Autodesk Inventor part; units mm, degrees
ref_plane "YZ Plane" through (0, 0, 0) normal (1, 0, 0) x (0, 1, 0)
ref_plane "XZ Plane" through (0, 0, 0) normal (0, 1, 0) x (-1, 0, 0)
ref_plane "XY Plane" through (0, 0, 0) normal (0, 0, 1) x (1, 0, 0)
sketch "Sketch1" plane through (0, 0, 0) normal (0, 0, 1) x (1, 0, 0)
  line L0 (0, 0) -> (0, 10)
  line L1 (0, 10) -> (-3, 10)
  line L2 (-3, 10) -> (-3, 20)
  line L3 (-3, 20) -> (0, 20)
  line L4 (0, 20) -> (0, 30)
  line L5 (0, 30) -> (38.5, 30)
  line L6 (38.5, 30) -> (38.5, 33)
  line L7 (38.5, 33) -> (48.5, 33)
  line L8 (48.5, 33) -> (48.5, 30)
  line L9 (48.5, 30) -> (87, 30)
  line L10 (87, 30) -> (87, 20)
  line L11 (87, 20) -> (90, 20)
  line L12 (90, 20) -> (90, 10)
  line L13 (90, 10) -> (87, 10)
  line L14 (87, 10) -> (87, 0)
  line L15 (87, 0) -> (48.5, 0)
  line L16 (48.5, 0) -> (48.5, -3)
  line L17 (48.5, -3) -> (38.5, -3)
  line L18 (38.5, -3) -> (38.5, 0)
  line L19 (38.5, 0) -> (0, 0)
  line L20 (10, 25) -> (20, 25)
  line L21 (25, 20) -> (25, 10)
  line L22 (20, 5) -> (10, 5)
  line L23 (5, 10) -> (5, 20)
  line L24 (67, 25) -> (77, 25)
  line L25 (82, 20) -> (82, 10)
  line L26 (77, 5) -> (67, 5)
  line L27 (62, 10) -> (62, 20)
  arc A0 (10, 25) -> (5, 20) centre (10, 20) ccw
  arc A1 (25, 20) -> (20, 25) centre (20, 20) ccw
  arc A2 (20, 5) -> (25, 10) centre (20, 10) ccw
  arc A3 (5, 10) -> (10, 5) centre (10, 10) ccw
  arc A4 (67, 25) -> (62, 20) centre (67, 20) ccw
  arc A5 (82, 20) -> (77, 25) centre (77, 20) ccw
  arc A6 (77, 5) -> (82, 10) centre (77, 10) ccw
  arc A7 (62, 10) -> (67, 5) centre (67, 10) ccw
  circle A8 centre (43.5, 15) radius 2.5
  circle A9 centre (35.3683, 23.1317) radius 1
  circle A10 centre (35.3683, 6.8683) radius 1
  circle A11 centre (51.6317, 6.8683) radius 1
  circle A12 centre (51.6317, 23.1317) radius 1
  dimension "d0" = 10
  dimension "d1" = 10
  dimension "d2" = 10
  dimension "d3" = 10
  dimension "d4" = 10
  dimension "d5" = 10
  dimension "d6" = 38.5
  dimension "d7" = 38.5
  dimension "d8" = 10
  dimension "d9" = 38.5
  dimension "d11" = 38.5
  dimension "d12" = 5
  dimension "d13" = 5
  dimension "d15" = 5
  dimension "d16" = 20
  dimension "d17" = 5
  dimension "d18" = 5
  dimension "d19" = 5
  dimension "d20" = 20
  dimension "d21" = 3
  dimension "d23" = 3
  dimension "d24" = 3
  dimension "d25" = 5
  dimension "d26" = 5
  dimension "d27" = 5
  dimension "d28" = 15
  dimension "d30" = 2
  dimension "d34" = 360
  dimension "d38" = 3
  dimension "d39" = 10
extrude "Extrusion1" add sketch "Sketch1" along normal blind 3
properties part number "OpenROV 2_3 Dev Vertical Motor Mount"
Geometry: final body of the model. Coordinates: model frame, mm. A direction names the side the tool comes from. Coordinates: 2 decimals unless noted, no trailing zeros. Order: outer loops, then holes, each group sorted by start corner. A loop starts at its lowest first (then second) coordinate and runs counter-clockwise, first axis right, second up.
Item 1: Material intervals for line 1 along Y through (x, z) = (51.5, 2.3); line 2 along X through (y, z) = (11.5, 0.8); line 3 along Y through (x, z) = (74.5, 1.7), sorted ascending.
Answer:
line 1: y = 0 to 5.88, 7.86 to 22.14, 24.12 to 30
line 2: x = -3 to 5, 25 to 62, 82 to 90
line 3: y = 0 to 5, 25 to 30
Item 2: Section query C-C (y = 9). Output: boundary loops of the cut face in (x, z), then the cut area to 3 significant figures.
Answer:
outline: (0, 0) - (5.1, 0) - (5.1, 3) - (0, 3) - close; (24.9, 0) - (62.1, 0) - (62.1, 3) - (24.9, 3) - close; (81.9, 0) - (87, 0) - (87, 3) - (81.9, 3) - close
area: 142 mm2
Item 3: Section query A-A (y = 15). Output: boundary loops of the cut face in (x, z), then the cut area to 3 significant figures.
Answer:
outline: (-3, 0) - (5, 0) - (5, 3) - (-3, 3) - close; (25, 0) - (41, 0) - (41, 3) - (25, 3) - close; (46, 0) - (62, 0) - (62, 3) - (46, 3) - close; (82, 0) - (90, 0) - (90, 3) - (82, 3) - close
area: 144 mm2
Item 4: Contact query for flat-ended pins moving along their axis: P1, Ø2.5, axis at x = 51.63, y = 23.13, coming from the +Z side; P2, Ø12, axis at x = 75, y = 15.5, coming from the -Z side; P3, Ø0.9, axis at x = -1.5, z = 1.5, coming from the +Y side; P4, Ø1.5, axis at y = 25, z = 1, coming from the -X side. Output: stop coordinate, or through.
Answer:
P1: stops at z = 3
P2: passes through
P3: stops at y = 20
P4: stops at x = 0
Item 5: Section query B-B (x = 73.5). Output: boundary loops of the cut face in (y, z), then the cut area to 3 significant figures.
Answer:
outline: (0, 0) - (5, 0) - (5, 3) - (0, 3) - close; (25, 0) - (30, 0) - (30, 3) - (25, 3) - close
area: 30.0 mm2
Item 6: Section query D-D (x = 43.5). Output: boundary loops of the cut face in (y, z), then the cut area to 3 significant figures.
Answer:
outline: (-3, 0) - (12.5, 0) - (12.5, 3) - (-3, 3) - close; (17.5, 0) - (33, 0) - (33, 3) - (17.5, 3) - close
area: 93.0 mm2
Item 7: Access query for faces 5 (the face through (89, 10, 1)), 6 (the face through (0, 5, 1)), 7 (the face through (24, 7, 1)). Directions: +Z, -Z, +X, -X, +Y, -Y. A direction counts if a zero-diameter tool reaches every point of the face in a straight line with its end or side. Return the directions, or none.
Answer:
face 5: +Z, -Z, +X, -Y
face 6: +Z, -Z, -X, -Y
face 7: +Z, -Z
Item 8: Draft query along X for faces 1 (the face through (72, 5, 1)), 2 (the face through (0, 25, 1)), 3 (the face through (-1, 10, 1)), 4 (the face through (52.586, 6.568, 1.479)). Return one class per face: released by +X, released by -X, zero draft, split by the parting line, or undercut.
Answer:
face 1: undercut
face 2: released by -X
face 3: zero draft
face 4: undercut
